Here's how the part is built. I have some questions about the finished solid (model axes, mm). A direction names the side the tool comes from. Coordinates: 2 decimals unless noted, no trailing zeros. Loops run counter-clockwise (first coordinate to the right, second up) from the corner with the lowest first, then second, coordinate; pieces in that order, holes last. Notation, with made-up numbers: M 37.25,43 L 65.25,43 A13 ccw 65.25,65 Z; hole C -4.75,29.25 d9. An arc over 180 degrees is marked long. Use CSV: the item, a comma, the result in double quotes. Start each with the question number.
Q1. For pin 1 Ø0.6 at (x, z) = (35.5, 36.5) entering from +Y; pin 2 Ø5 at (y, z) = (15.5, 14.5) entering from +X; pin 3 Ø8 at (x, y) = (17.5, 37.5) entering from +Z, each with a flat end and sliding along its axis, tell me the tip position at first contact or that it passes through.
Q2. If we section it at D-D (z = 35.5): Please give me the cut outline in (x, y).
Q3. If we section it at B-B (z = 29): Please give me the cut outline in (x, y), and give its area (3 significant figures).
Q4. Please list where these lines run through material, in increasing order: probe 1 along X at (y, z) = (8, 3); probe 2 along X at (y, z) = (10, 9.5); probe 3 along X at (y, z) = (33.5, 33). Write a range as [from, to].
Q5. If we section it at A-A (x = 8): Please give me the cut outline in (y, z), and give its area (3 significant figures).
Q6. Which directions (+Z, -Z, +X, -X, +Y, -Y) give clear straight access to the entire face, cutting with the end or side of a thin tool? Please do faces 1 (the flat face through (47.095, 25.329, 0.761)), 2 (the flat face through (23.595, 49.26, 3.365)), 3 (the flat face through (35, 25, 36.995)), 4 (the flat face through (34.295, 25, 36)).
Q7. If we mould it in two halves opening along X, with no side actions, what happens to faces 5 (the flat face through (13.1, 0.7, 0.8)), 6 (the flat face through (67.12, 24.66, 0.74)), 7 (the flat face through (43.18, 24.67, 7.73))? For each: +X half, -X half, draft (parallel to the pull), parting line (faces both ways), or undercut.
Q8. If we section it at C-C (y = 20): Please give me the cut outline in (x, z), and give its area (3 significant figures).
from build123d import *
from OCP.BRepFilletAPI import BRepFilletAPI_MakeChamfer

# Parameters (mm, degrees)
BOSS_EXTRUDE1_DEPTH = 50
CUT_EXTRUDE3_DEPTH  = 94.541434669
CHAMFER2_SIZE       = 4
CHAMFER2_SIZE2      = 2.828427125
CHAMFER3_SIZE       = 1.5
CHAMFER4_SIZE       = 1.5
SKETCH6_W           = 2.121320343
SKETCH6_H           = 7
BOSS_EXTRUDE2_DEPTH = 7
SKETCH7_W           = 1.8
SKETCH7_H           = 1.8
CUT_EXTRUDE4_DEPTH  = 7


with BuildPart() as part:
    # Sketch4 → Boss-Extrude1 (new body)
    with BuildSketch(Plane(origin=(0, 0, 0), x_dir=(1, 0, 0), z_dir=(0, 1, 0))):
        Polygon((0, 0), (70.710678119, 0), (35.355339059, -35.355339059), align=None)
    extrude(amount=BOSS_EXTRUDE1_DEPTH)

    # Sketch5 → Cut-Extrude3 (cut, through all)
    with BuildSketch(Plane.XZ):
        Polygon((39.911688245, 11), (30.798989873, 11), (24.355339059, 4.556349186), (24.355339059, -4.556349186), (30.798989873, -11), (39.911688245, -11), (46.355339059, -4.556349186), (46.355339059, 4.556349186), align=None)
    extrude(amount=-CUT_EXTRUDE3_DEPTH, mode=Mode.SUBTRACT)

    # Chamfer2: one chamfer whose edges measure the first distance from different faces: ONE call of the kernel's chamfer builder (chamfer() names one face for all edges)
    chamfer2_edges_1 = [part.edges().sort_by_distance(p)[0] for p in [
        (0, 25, 0),
    ]]
    chamfer2_side_1 = [part.faces().sort_by_distance(p)[0] for p in [
        (17.67766953, 25, 17.67766953),
    ]]
    chamfer2_edges_2 = [part.edges().sort_by_distance(p)[0] for p in [
        (70.710678119, 25, 0),
    ]]
    chamfer2_side_2 = [part.faces().sort_by_distance(p)[0] for p in [
        (53.033008589, 25, 17.67766953),
    ]]
    chamfer2 = BRepFilletAPI_MakeChamfer(part.part.solid().wrapped)
    for e in chamfer2_edges_1:
        chamfer2.Add(CHAMFER2_SIZE, CHAMFER2_SIZE2, e.wrapped, chamfer2_side_1[0].wrapped)  # the first distance lies on this face
    for e in chamfer2_edges_2:
        chamfer2.Add(CHAMFER2_SIZE, CHAMFER2_SIZE2, e.wrapped, chamfer2_side_2[0].wrapped)  # the first distance lies on this face
    add(Compound.cast(chamfer2.Shape()), mode=Mode.REPLACE)

    # Chamfer3
    chamfer3_edges = [part.edges().sort_by_distance(p)[0] for p in [
        (13.591883092, 0, 0),
        (46.355339059, 0, 2.278174593),
        (13.591883092, 50, 0),
        (24.355339059, 0, 2.278174593),
        (43.133513652, 0, 7.778174593),
        (27.577164466, 0, 7.778174593),
        (46.355339059, 25, 0),
        (46.355339059, 50, 2.278174593),
        (24.355339059, 50, 2.278174593),
        (24.355339059, 25, 0),
        (43.133513652, 50, 7.778174593),
        (27.577164466, 50, 7.778174593),
        (57.118795027, 0, 0),
        (2.828427125, 25, 0),
        (57.118795027, 50, 0),
        (67.882250994, 25, 0),
        (35.355339059, 25, 35.355339059),
    ]]
    chamfer(chamfer3_edges, length=CHAMFER3_SIZE)

    # Chamfer4
    chamfer4_edges = [part.edges().sort_by_distance(p)[0] for p in [
        (18.561553006, 0, 18.561553006),
        (18.561553006, 50, 18.561553006),
        (2.828427125, 0, 2.164213562),
        (67.882250994, 50, 2.164213562),
        (2.828427125, 50, 2.164213562),
        (52.149125113, 50, 18.561553006),
        (35.355339059, 50, 34.294678888),
        (67.882250994, 0, 2.164213562),
        (52.149125113, 0, 18.561553006),
        (35.355339059, 0, 34.294678888),
    ]]
    chamfer(chamfer4_edges, length=CHAMFER4_SIZE)

    # Sketch6 → Boss-Extrude2 (add)
    with BuildSketch(Plane.XY.offset(34.294678888)):
        with Locations((35.355339059, 25)):
            Rectangle(SKETCH6_W, SKETCH6_H)
    extrude(amount=BOSS_EXTRUDE2_DEPTH)

    # Sketch7 → Cut-Extrude4 (cut)
    with BuildSketch(Plane(origin=(36.415999231, 0, 0), x_dir=(0, 0, -1), z_dir=(1, 0, 0))):
        with Locations((-37.894678888, 25)):
            Rectangle(SKETCH7_W, SKETCH7_H)
    extrude(amount=-CUT_EXTRUDE4_DEPTH, mode=Mode.SUBTRACT)


solid = part.part
Results below:
1,pin 1,"y = 28.5"
1,pin 2,"x = 58.71"
1,pin 3,"z = 21.5"
2,outline,"M 34.29,21.5 L 36.42,21.5 L 36.42,28.5 L 34.29,28.5 Z"
3,outline,"M 29,1.5 L 31.12,0 L 39.59,0 L 41.71,1.5 L 41.71,48.5 L 39.59,50 L 31.12,50 L 29,48.5 Z"
3,area,"629 mm^2"
4,probe 1,"[3, 24.36], [46.36, 67.71]"
4,probe 2,"[9.5, 29.3], [41.41, 61.21]"
4,probe 3,"[33, 37.71]"
5,outline,"M 0,1.5 L 1.5,0 L 48.5,0 L 50,1.5 L 50,5.88 L 48.5,8 L 1.5,8 L 0,5.88 Z"
5,area,"395 mm^2"
6,face 1,"-Z, +Y, -Y"
6,face 2,"-Z, +Y"
6,face 3,"+X, -X"
6,face 4,"+Z, -X, +Y, -Y"
7,face 5,"draft"
7,face 6,"+X half"
7,face 7,"undercut"
8,outline,"M 2.83,1.5 L 4.33,0 L 22.86,0 L 24.36,1.5 L 24.36,4.56 L 30.8,11 L 39.91,11 L 46.36,4.56 L 46.36,1.5 L 47.86,0 L 66.38,0 L 67.88,1.5 L 67.88,2.83 L 36.42,34.29 L 34.29,34.29 L 2.83,2.83 Z"
8,area,"1,040 mm^2"
